Autodesk Inventor part; units mm, degrees
ref_plane "YZ Plane" through (0, 0, 0) normal (1, 0, 0) x (0, 1, 0)
ref_plane "XZ Plane" through (0, 0, 0) normal (0, 1, 0) x (-1, 0, 0)
ref_plane "XY Plane" through (0, 0, 0) normal (0, 0, 1) x (1, 0, 0)
sketch "Boceto1" plane through (0, 0, 0) normal (0, 0, 1) x (1, 0, 0)
  line L0 (0, 3) -> (170, 3)
  line L1 (0, 113) -> (170, 113)
  line L2 (10, 103) -> (10, 13)
  line L3 (10, 13) -> (160, 13)
  line L4 (160, 13) -> (160, 103)
  line L5 (10, 103) -> (160, 103)
  line L6 (85, 169.6763) -> (0, 113)
  line L7 (85, 169.6763) -> (170, 113)
  line L8 (0, 92.5) -> (0, 107.7321)
  line L9 (0, 92.5) -> (3, 92.5)
  line L10 (3, 107.7321) -> (3, 92.5)
  line L11 (0, 107.7321) -> (3, 107.7321)
  line L12 (3, 113) -> (3, 107.7321)
  line L13 (3, 92.5) -> (3, 78.5)
  line L14 (0, 65) -> (0, 78.5)
  line L15 (0, 65) -> (3, 65)
  line L16 (3, 78.5) -> (3, 65)
  line L17 (0, 78.5) -> (3, 78.5)
  line L18 (3, 65) -> (3, 51)
  line L19 (0, 37.5) -> (0, 51)
  line L20 (0, 37.5) -> (3, 37.5)
  line L21 (3, 51) -> (3, 37.5)
  line L22 (0, 51) -> (3, 51)
  line L23 (3, 37.5) -> (3, 23.5)
  line L24 (0, 10) -> (0, 23.5)
  line L25 (0, 10) -> (3, 10)
  line L26 (3, 23.5) -> (3, 10)
  line L27 (0, 23.5) -> (3, 23.5)
  line L28 (3, 10) -> (3, 3)
  line L29 (170, 113) -> (170, 107.7321)
  line L30 (170, 113) -> (167, 113)
  line L31 (167, 107.7321) -> (167, 113)
  line L32 (170, 107.7321) -> (167, 107.7321)
  line L33 (167, 92.5) -> (167, 107.7321)
  line L34 (170, 92.5) -> (170, 78.5)
  line L35 (170, 92.5) -> (167, 92.5)
  line L36 (167, 78.5) -> (167, 92.5)
  line L37 (170, 78.5) -> (167, 78.5)
  line L38 (167, 65) -> (167, 78.5)
  line L39 (170, 65) -> (170, 51)
  line L40 (170, 65) -> (167, 65)
  line L41 (167, 51) -> (167, 65)
  line L42 (170, 51) -> (167, 51)
  line L43 (167, 37.5) -> (167, 51)
  line L44 (170, 37.5) -> (170, 23.5)
  line L45 (170, 37.5) -> (167, 37.5)
  line L46 (167, 23.5) -> (167, 37.5)
  line L47 (170, 23.5) -> (167, 23.5)
  line L48 (167, 8.2679) -> (167, 23.5)
  line L49 (170, 8.2679) -> (170, 3)
  line L50 (170, 8.2679) -> (167, 8.2679)
  line L51 (167, 3) -> (167, 8.2679)
  line L52 (170, 3) -> (167, 3)
  point P0 (0, 0)
  point P1 (86.5, 171.1763)
  point P2 (83.5, 171.1763)
  dimension "d0" = 110
  dimension "d8" = 10
extrude "Extrusión1" add sketch "Boceto1" against normal blind 3
Build history of the part. All positions in model axes, mm. Round coordinates to 2 decimals unless told otherwise and drop trailing zeros. Write each loop counter-clockwise with the first axis right and the second up, starting at its lowest first coordinate (ties: lowest second). Pieces come first, ordered by that corner, then holes.
1) Band-saw the part on A-A, the plane y = 99.5. List the corners of the cut face in (x, z).
2) Band-saw the part on C-C, the plane y = 139.5. List the corners of the cut face in (x, z).
3) Pin check, flat tips, straight feed: pin 1 (1 mm diameter, centred on y = 87.5, z = -2, fed in from -X); pin 2 (1.5 mm diameter, centred on x = 1.5, z = -1, fed in from +Y); pin 3 (1.5 mm diameter, centred on x = 169, z = -1.5, fed in from +Y). Stop position of each tip, or through.
4) Band-saw the part on B-B, the plane x = 27.5. List the corners of the cut face in (y, z).
5) Drill centre lines: probe 1 along X at (y, z) = (50, -2.05); probe 2 along X at (y, z) = (51.5, -1.45); probe 3 along Y at (x, z) = (60, -0.65). Where is each one in solid material? Low to high.
6) Band-saw the part on D-D, the plane y = 122.5. List the corners of the cut face in (x, z), and give its area (3 significant figures).
Ans:
1. outline: (0, -3) - (10, -3) - (10, 0) - (0, 0) - close; (160, -3) - (167, -3) - (167, 0) - (160, 0) - close
2. outline: (39.74, -3) - (130.26, -3) - (130.26, 0) - (39.74, 0) - close
3. pin 1: stops at x = 3
3. pin 2: stops at y = 114.5
3. pin 3: stops at y = 114.17
4. outline: (3, -3) - (13, -3) - (13, 0) - (3, 0) - close; (103, -3) - (131.34, -3) - (131.34, 0) - (103, 0) - close
5. probe 1: x = 0 to 10, 160 to 167
5. probe 2: x = 3 to 10, 160 to 170
5. probe 3: y = 3 to 13, 103 to 153.01
6. outline: (14.25, -3) - (155.75, -3) - (155.75, 0) - (14.25, 0) - close
6. area: 425 mm2
